```python
from build123d import *

# Parameters (mm, degrees)
BOSS_EXTRUDE1_DEPTH = 1.5875


with BuildPart() as part:
    # Sketch1 → Boss-Extrude1 (new body)
    with BuildSketch(Plane.XY.offset(-447.675)):
        with BuildLine():
            Line((94.488, -85.725), (88.9, -85.725))
            Line((88.9, -85.725), (88.9, -60.325))
            Line((88.9, -60.325), (94.488, -60.325))
            Line((94.488, -60.325), (94.488, -26.162))
            ThreePointArc((94.488, -26.162), (87.048512242, -8.201487758), (69.088, -0.762))
            Line((69.088, -0.762), (-69.088, -0.762))
            ThreePointArc((-69.088, -0.762), (-87.048512242, -8.201487758), (-94.488, -26.162))
            Line((-94.488, -26.162), (-94.488, -60.325))
            Line((-94.488, -60.325), (-88.9, -60.325))
            Line((-88.9, -60.325), (-88.9, -85.725))
            Line((-88.9, -85.725), (-94.488, -85.725))
            Line((-94.488, -85.725), (-94.488, -111.125))
            Line((-94.488, -111.125), (-63.5, -111.125))
            Line((-63.5, -111.125), (-63.5, -114.3))
            Line((-63.5, -114.3), (-84.455, -114.3))
            ThreePointArc((-84.455, -114.3), (-85.353025612, -114.671974388), (-85.725, -115.57))
            Line((-85.725, -115.57), (-85.725, -136.525))
            Line((-85.725, -136.525), (-94.488, -136.525))
            Line((-94.488, -136.525), (-94.488, -170.688))
            ThreePointArc((-94.488, -170.688), (-87.048512242, -188.648512242), (-69.088, -196.088))
            Line((-69.088, -196.088), (69.088, -196.088))
            ThreePointArc((69.088, -196.088), (87.048512242, -188.648512242), (94.488, -170.688))
            Line((94.488, -170.688), (94.488, -136.525))
            Line((94.488, -136.525), (85.725, -136.525))
            Line((85.725, -136.525), (85.725, -115.57))
            ThreePointArc((85.725, -115.57), (85.353025612, -114.671974388), (84.455, -114.3))
            Line((84.455, -114.3), (63.5, -114.3))
            Line((63.5, -114.3), (63.5, -111.125))
            Line((63.5, -111.125), (94.488, -111.125))
            Line((94.488, -111.125), (94.488, -85.725))
        make_face()
        with BuildLine():
            Line((-48.874039546, -127), (-34.925, -127))
            ThreePointArc((-34.925, -127), (-30.434871939, -128.859871939), (-28.575, -133.35))
            Line((-28.575, -133.35), (-28.575, -180.213))
            ThreePointArc((-28.575, -180.213), (-30.434871939, -184.703128061), (-34.925, -186.563))
            Line((-34.925, -186.563), (-59.563, -186.563))
            ThreePointArc((-59.563, -186.563), (-61.993039796, -186.079635031), (-64.053128061, -184.703128061))
            Line((-64.053128061, -184.703128061), (-82.140147834, -166.616108288))
            ThreePointArc((-82.140147834, -166.616108288), (-84.000019773, -162.125980227), (-82.140147834, -157.635852166))
            Line((-82.140147834, -157.635852166), (-53.364167607, -128.859871939))
            ThreePointArc((-53.364167607, -128.859871939), (-51.304079342, -127.483364969), (-48.874039546, -127))
        make_face(mode=Mode.SUBTRACT)
        with BuildLine():
            Line((28.575, -133.35), (28.575, -180.213))
            ThreePointArc((28.575, -180.213), (30.434871939, -184.703128061), (34.925, -186.563))
            Line((34.925, -186.563), (69.088, -186.563))
            ThreePointArc((69.088, -186.563), (80.313320151, -181.913320151), (84.963, -170.688))
            Line((84.963, -170.688), (84.963, -163.088960454))
            ThreePointArc((84.963, -163.088960454), (84.479635031, -160.658920658), (83.103128061, -158.598832393))
            Line((83.103128061, -158.598832393), (53.364167607, -128.859871939))
            ThreePointArc((53.364167607, -128.859871939), (51.304079342, -127.483364969), (48.874039546, -127))
            Line((48.874039546, -127), (34.925, -127))
            ThreePointArc((34.925, -127), (30.434871939, -128.859871939), (28.575, -133.35))
        make_face(mode=Mode.SUBTRACT)
        with BuildLine():
            Line((-12.7, -127), (12.7, -127))
            ThreePointArc((12.7, -127), (17.190128061, -128.859871939), (19.05, -133.35))
            Line((19.05, -133.35), (19.05, -180.213))
            ThreePointArc((19.05, -180.213), (17.190128061, -184.703128061), (12.7, -186.563))
            Line((12.7, -186.563), (-12.7, -186.563))
            ThreePointArc((-12.7, -186.563), (-17.190128061, -184.703128061), (-19.05, -180.213))
            Line((-19.05, -180.213), (-19.05, -133.35))
            ThreePointArc((-19.05, -133.35), (-17.190128061, -128.859871939), (-12.7, -127))
        make_face(mode=Mode.SUBTRACT)
        with BuildLine():
            Line((-84.963, -26.162), (-84.963, -43.671231637))
            ThreePointArc((-84.963, -43.671231637), (-84.479635031, -46.101271432), (-83.103128061, -48.161359697))
            Line((-83.103128061, -48.161359697), (-70.401634909, -60.862852849))
            ThreePointArc((-70.401634909, -60.862852849), (-68.341546644, -62.23935982), (-65.911506848, -62.722724789))
            Line((-65.911506848, -62.722724789), (-25.898012242, -62.722724789))
            ThreePointArc((-25.898012242, -62.722724789), (-22.964694726, -60.762744686), (-23.652948212, -57.302660758))
            Line((-23.652948212, -57.302660758), (-68.129730486, -12.825878484))
            ThreePointArc((-68.129730486, -12.825878484), (-71.341107932, -11.096095222), (-74.974430911, -11.418677575))
            ThreePointArc((-74.974430911, -11.418677575), (-82.230730228, -17.257828666), (-84.963, -26.162))
        make_face(mode=Mode.SUBTRACT)
        with BuildLine():
            Line((-49.461238683, -10.358858045), (-11.1125, -10.358858045))
            ThreePointArc((-11.1125, -10.358858045), (-6.622371939, -12.218729985), (-4.7625, -16.708858045))
            Line((-4.7625, -16.708858045), (-4.7625, -55.057596728))
            ThreePointArc((-4.7625, -55.057596728), (-6.722480102, -57.990914244), (-10.18256403, -57.302660758))
            Line((-10.18256403, -57.302660758), (-51.706302713, -15.778922075))
            ThreePointArc((-51.706302713, -15.778922075), (-52.394556199, -12.318838147), (-49.461238683, -10.358858045))
        make_face(mode=Mode.SUBTRACT)
        with BuildLine():
            Line((4.7625, -16.708858045), (4.7625, -55.057596728))
            ThreePointArc((4.7625, -55.057596728), (6.722480102, -57.990914244), (10.18256403, -57.302660758))
            Line((10.18256403, -57.302660758), (51.706302713, -15.778922075))
            ThreePointArc((51.706302713, -15.778922075), (52.394556199, -12.318838147), (49.461238683, -10.358858045))
            Line((49.461238683, -10.358858045), (11.1125, -10.358858045))
            ThreePointArc((11.1125, -10.358858045), (6.622371939, -12.218729985), (4.7625, -16.708858045))
        make_face(mode=Mode.SUBTRACT)
        with BuildLine():
            Line((68.129730486, -12.825878484), (23.652948212, -57.302660758))
            ThreePointArc((23.652948212, -57.302660758), (22.964694726, -60.762744686), (25.898012242, -62.722724789))
            Line((25.898012242, -62.722724789), (65.911506848, -62.722724789))
            ThreePointArc((65.911506848, -62.722724789), (68.341546644, -62.23935982), (70.401634909, -60.862852849))
            Line((70.401634909, -60.862852849), (83.103128061, -48.161359697))
            ThreePointArc((83.103128061, -48.161359697), (84.479635031, -46.101271432), (84.963, -43.671231637))
            Line((84.963, -43.671231637), (84.963, -26.162))
            ThreePointArc((84.963, -26.162), (82.230730228, -17.257828666), (74.974430911, -11.418677575))
            ThreePointArc((74.974430911, -11.418677575), (71.341107932, -11.096095222), (68.129730486, -12.825878484))
        make_face(mode=Mode.SUBTRACT)
        with BuildLine():
            Line((68.383887592, -125.919079683), (72.874015653, -130.409207744))
            ThreePointArc((72.874015653, -130.409207744), (72.874015653, -134.899335804), (68.383887592, -134.899335804))
            Line((68.383887592, -134.899335804), (63.893759532, -130.409207744))
            ThreePointArc((63.893759532, -130.409207744), (63.893759532, -125.919079683), (68.383887592, -125.919079683))
        make_face(mode=Mode.SUBTRACT)
        with BuildLine():
            Line((-80.313320151, -177.423192091), (-75.823192091, -181.913320151))
            ThreePointArc((-75.823192091, -181.913320151), (-75.823192091, -186.403448212), (-80.313320151, -186.403448212))
            Line((-80.313320151, -186.403448212), (-84.803448212, -181.913320151))
            ThreePointArc((-84.803448212, -181.913320151), (-84.803448212, -177.423192091), (-80.313320151, -177.423192091))
        make_face(mode=Mode.SUBTRACT)
    extrude(amount=-BOSS_EXTRUDE1_DEPTH)


solid = part.part
```
Input: part model. Units: mm. Frame: model coordinates. Give positions to 0.01 mm unless a question says otherwise; leave off trailing zeros. Loops run counter-clockwise (first coordinate to the right, second up) from the corner with the lowest first, then second, coordinate; pieces in that order, holes last.
1) Contact query for flat-ended pins moving along their axis: pin 1 (0.5 mm diameter, centred on y = -69, z = -448.5, fed in from +X); pin 2 (0.5 mm diameter, centred on x = 92, z = -449, fed in from +Y). Output: stop coordinate, or through.
A:
pin 1: stops at x = 88.9
pin 2: stops at y = -14.69
2) Line query: L1, parallel to Y at x = 5.5, z = -448; L2, parallel to X at y = -45, z = -447.75; L3, parallel to X at y = -178.5, z = -448.5 (3 decimals). Output: solid intervals per line, ascending.
A:
L1: y = -196.09 to -186.56, -127 to -57.09, -13.74 to -0.76
L2: x = -94.49 to -84.82, -35.96 to -22.49, -4.76 to 4.76, 22.49 to 35.96, 84.82 to 94.49
L3: x = -93.257 to -85.511, -79.237 to -70.256, -28.575 to -19.05, 19.05 to 28.575, 82.908 to 93.257
3) Section query D-D on y = -77. Return the cut outline in (x, z) (1 decimal), and give its area (3 significant figures).
A:
outline: (-88.9, -449.3) - (88.9, -449.3) - (88.9, -447.7) - (-88.9, -447.7) - close
area: 282 mm2
4) Mould query, pull axis Y, two halves, no side actions, for faces 1 (the flat face through (-1, -97, -449.262)), 2 (the cylindrical face through (-86.85, -8.005, -448.458)), 3 (the cylindrical face through (63.845, -125.969, -448.458)), 4 (the cylindrical face through (86.85, -188.845, -448.458)). Classes: released by +Y, released by -Y, zero draft, split by the parting line, or undercut.
A:
face 1: zero draft
face 2: released by +Y
face 3: undercut
face 4: released by -Y
5) Section query B-B on y = -153. Count the separate pieces of the cut face and the enclosed holes in it, and give its area (3 significant figures).
A:
separate pieces: 4
enclosed holes: 0
area: 84.2 mm2
6) Section query A-A on y = -20.5. Return the cut outline in (x, z) (1 decimal), and give its area (3 significant figures).
A:
outline: (-93.8, -449.3) - (-83.9, -449.3) - (-83.9, -447.7) - (-93.8, -447.7) - close; (-60.5, -449.3) - (-47, -449.3) - (-47, -447.7) - (-60.5, -447.7) - close; (-4.8, -449.3) - (4.8, -449.3) - (4.8, -447.7) - (-4.8, -447.7) - close; (47, -449.3) - (60.5, -449.3) - (60.5, -447.7) - (47, -447.7) - close; (83.9, -449.3) - (93.8, -449.3) - (93.8, -447.7) - (83.9, -447.7) - close
area: 89.4 mm2
